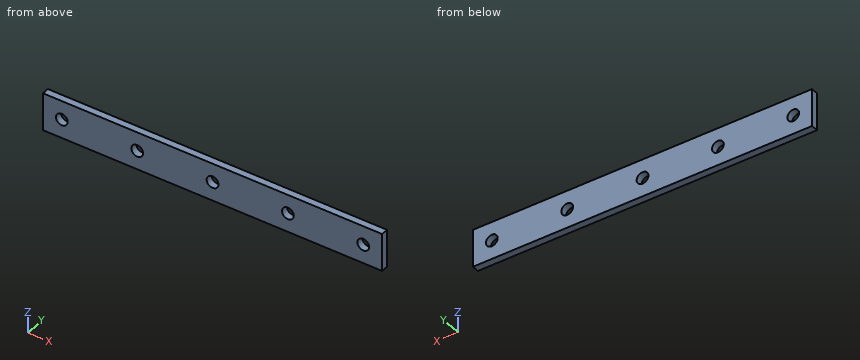
from build123d import *

# Parameters (mm, degrees)
F0_W     = 144
F0_H     = 16
F0_R     = 2.5
F1_DEPTH = 3


with BuildPart() as f1:
    # F0 (on Front) → F1 (new body)
    with BuildSketch(Plane.XZ):
        Rectangle(F0_W, F0_H)
        with Locations((-64, 0)):
            Circle(F0_R, mode=Mode.SUBTRACT)
        with Locations((-32, 0)):
            Circle(F0_R, mode=Mode.SUBTRACT)
        Circle(F0_R, mode=Mode.SUBTRACT)
        with Locations((32, 0)):
            Circle(F0_R, mode=Mode.SUBTRACT)
        with Locations((64, 0)):
            Circle(F0_R, mode=Mode.SUBTRACT)
    extrude(amount=F1_DEPTH)


solid = f1.part
Geometry check sheet. Reference: the model listing, model coordinates, mm. Round coordinates to 2 decimals unless told otherwise and drop trailing zeros. Order: outer loops, then holes, each group sorted by start corner. A loop starts at its lowest first (then second) coordinate and runs counter-clockwise, first axis right, second up. Notation, with made-up numbers: M -21,-31 L -15,-31 A21 ccw -15,-25 Z; hole C 71.25,49.5 d7. An arc over 180 degrees is marked long. Answer in a Markdown table with one row per item.
(1) Sectioned sample at B-B, the plane x = 64. Record the cut outline in (y, z).
Responses:
| item | result |
|---|---|
| outline | M -3,-8 L 0,-8 L 0,-2.5 L -3,-2.5 Z; M -3,2.5 L 0,2.5 L 0,8 L -3,8 Z |
(2) Sectioned sample at A-A, the plane z = 0. Record the cut outline in (x, y), and give its area (3 significant figures).
Responses:
| item | result |
|---|---|
| outline | M -72,-3 L -66.5,-3 L -66.5,0 L -72,0 Z; M -61.5,-3 L -34.5,-3 L -34.5,0 L -61.5,0 Z; M -29.5,-3 L -2.5,-3 L -2.5,0 L -29.5,0 Z; M 2.5,-3 L 29.5,-3 L 29.5,0 L 2.5,0 Z; M 34.5,-3 L 61.5,-3 L 61.5,0 L 34.5,0 Z; M 66.5,-3 L 72,-3 L 72,0 L 66.5,0 Z |
| area | 357 mm² |
(3) Sectioned sample at C-C, the plane y = -0.6. Record the cut outline in (x, z), and give its area (3 significant figures).
Responses:
| item | result |
|---|---|
| outline | M -72,-8 L 72,-8 L 72,8 L -72,8 Z; hole C -64,0 d5; hole C -32,0 d5; hole C 0,0 d5; hole C 32,0 d5; hole C 64,0 d5 |
| area | 2,210 mm² |
(4) Scan lines: probe 1 along Z at (x, y) = (-64, -0.9); probe 2 along X at (y, z) = (-2.1, -2); probe 3 along Z at (x, y) = (-30.5, -0.3). Record each from-to range of solid material in increasing order. Write a range as from..to.
Responses:
| item | result |
|---|---|
| probe 1 | z = -8..-2.5, 2.5..8 |
| probe 2 | x = -72..-65.5, -62.5..-33.5, -30.5..-1.5, 1.5..30.5, 33.5..62.5, 65.5..72 |
| probe 3 | z = -8..-2, 2..8 |
